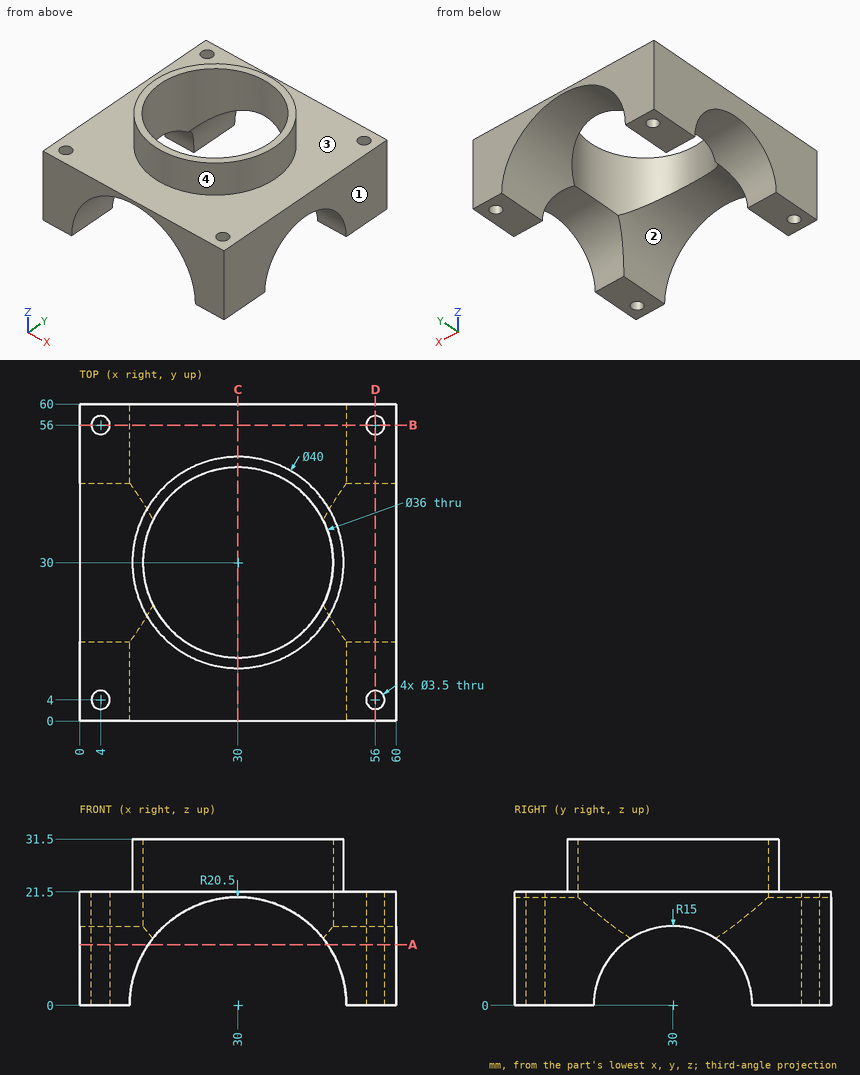
Check sheet for the drawn part. Datum: minimum x, y, z corner. Units: mm. Give positions to 0.01 mm unless a question says otherwise; leave off trailing zeros. Write each loop counter-clockwise with the first axis right and the second up, starting at its lowest first coordinate (ties: lowest second). Pieces come first, ordered by that corner, then holes. Notation, with made-up numbers: (57, -6.5) - (67, -6.5) arc R26 cw to (67, 19.5) - close; hole circle Ø8 at (-19, 85.25). An arc over 180 degrees is marked (long way). Put each result on its own line as item: value.
1. Sectioned sample at D-D, the plane x = 56. Enter the section's corners in (y, z), plus the area to 3 significant figures.
Ans:
outline: (0, 0) - (2.25, 0) - (2.25, 21.5) - (0, 21.5) - close; (5.75, 0) - (15, 0) arc R15 cw to (45, 0) - (54.25, 0) - (54.25, 21.5) - (5.75, 21.5) - close; (57.75, 0) - (60, 0) - (60, 21.5) - (57.75, 21.5) - close
area: 786 mm²
2. Draft check along X on the marked faces 1, 2, 3 and 4. Enter one of: +X half, -X half, draft (parallel to the pull), parting line (faces both ways), or undercut.
Ans:
face 1: +X half
face 2: undercut
face 3: draft
face 4: parting line
3. Go/stop test with a flat-tipped pin: pin 1 (2 mm diameter, centred on y = 49, z = 27, fed in from -X). Record where the tip stops, or that it passes through.
Ans:
pin 1: stops at x = 21.28
4. Thickness scan on line 1 (X direction, y = 29.5, z = 22.5); line 2 (Y direction, x = 5, z = 16); line 3 (Y direction, x = 30, z = 24.5). Record the ranges inside material, lowest first.
Ans:
line 1: x = 10.01 to 12.01, 47.99 to 49.99
line 2: y = 0 to 2.56, 5.44 to 54.56, 57.44 to 60
line 3: y = 10 to 12, 48 to 50
5. Sectioned sample at C-C, the plane x = 30. Enter the section's corners in (y, z), plus the area to 3 significant figures.
Ans:
outline: (0, 20.5) - (12, 20.5) - (12, 31.5) - (10, 31.5) - (10, 21.5) - (0, 21.5) - close; (48, 20.5) - (60, 20.5) - (60, 21.5) - (50, 21.5) - (50, 31.5) - (48, 31.5) - close
area: 64.0 mm²
6. Sectioned sample at B-B, the plane y = 56. Enter the section's corners in (x, z), plus the area to 3 significant figures.
Ans:
outline: (0, 0) - (2.25, 0) - (2.25, 21.5) - (0, 21.5) - close; (5.75, 0) - (9.5, 0) arc R20.5 cw to (50.5, 0) - (54.25, 0) - (54.25, 21.5) - (5.75, 21.5) - close; (57.75, 0) - (60, 0) - (60, 21.5) - (57.75, 21.5) - close
area: 479 mm²
7. Sectioned sample at A-A, the plane z = 11.5. Enter the section's corners in (x, y), plus the area to 3 significant figures.
Ans:
outline: (0, 0) - (13.03, 0) - (13.03, 20.37) - (0, 20.37) - close; (0, 39.63) - (13.03, 39.63) - (13.03, 60) - (0, 60) - close; (46.97, 0) - (60, 0) - (60, 20.37) - (46.97, 20.37) - close; (46.97, 39.63) - (60, 39.63) - (60, 60) - (46.97, 60) - close; hole circle Ø3.5 at (4, 4); hole circle Ø3.5 at (4, 56); hole circle Ø3.5 at (56, 4); hole circle Ø3.5 at (56, 56)
area: 1,020 mm²
